from build123d import *

# Parameters (mm, degrees)
SKETCH_1_R          = 1.25
SKETCH_1_R_2        = 4.8
EXTRUDE_1_DEPTH     = 2
SKETCH_3_R          = 6.5
SKETCH_3_R_2        = 4.8
EXTRUDE_2_DEPTH     = 2
SKETCH_5_R          = 1.25
CUT_EXTRUDE_1_DEPTH = 10


with BuildPart() as part:
    # 草图1 → 凸台-拉伸1 (new body)
    with BuildSketch(Plane(origin=(0, 0, 0), x_dir=(1, 0, 0), z_dir=(0, 1, 0))):
        with BuildLine():
            Line((10.5, -13.247031622), (-10.5, -13.247031622))
            ThreePointArc((-10.5, -13.247031622), (-14.742640687, -11.489672309), (-16.5, -7.247031622))
            Line((-16.5, -7.247031622), (-16.5, 7.247031622))
            ThreePointArc((-16.5, 7.247031622), (-14.742640687, 11.489672309), (-10.5, 13.247031622))
            Line((-10.5, 13.247031622), (10.5, 13.247031622))
            ThreePointArc((10.5, 13.247031622), (14.742640687, 11.489672309), (16.5, 7.247031622))
            Line((16.5, 7.247031622), (16.5, -7.247031622))
            ThreePointArc((16.5, -7.247031622), (14.742640687, -11.489672309), (10.5, -13.247031622))
        make_face()
        with Locations(Location((0, 8, 0), (0, 0, 270))):
            Circle(SKETCH_1_R, mode=Mode.SUBTRACT)
        with Locations(Location((0, -8, 0), (0, 0, 270))):
            Circle(SKETCH_1_R, mode=Mode.SUBTRACT)
        with Locations(Location((-9.5, 0, 0), (0, 0, 270))):
            Circle(SKETCH_1_R, mode=Mode.SUBTRACT)
        with Locations(Location((9.5, 0, 0), (0, 0, 270))):
            Circle(SKETCH_1_R, mode=Mode.SUBTRACT)
        with Locations(Location((0, 0, 0), (0, 0, 270))):
            Circle(SKETCH_1_R_2, mode=Mode.SUBTRACT)
    extrude(amount=EXTRUDE_1_DEPTH)

    # 草图3 → 凸台-拉伸2 (add)
    with BuildSketch(Plane(origin=(0, 2, 0), x_dir=(1, 0, 0), z_dir=(0, 1, 0))):
        with Locations(Location((0, 0, 0), (0, 0, 90))):
            Circle(SKETCH_3_R)
        with Locations(Location((0, 0, 0), (0, 0, 270))):
            Circle(SKETCH_3_R_2, mode=Mode.SUBTRACT)
    extrude(amount=EXTRUDE_2_DEPTH)

    # 草图5 → 切除-拉伸1 (cut)
    with BuildSketch(Plane(origin=(0, 2, 0), x_dir=(1, 0, 0), z_dir=(0, 1, 0))):
        with Locations(Location((-12.23, 2.77, 0), (0, 0, 270))):
            Circle(SKETCH_5_R)
        with Locations(Location((-12.23, -2.77, 0), (0, 0, 270))):
            Circle(SKETCH_5_R)
        with Locations(Location((12.23, -2.77, 0), (0, 0, 270))):
            Circle(SKETCH_5_R)
        with Locations(Location((12.23, 2.77, 0), (0, 0, 270))):
            Circle(SKETCH_5_R)
    extrude(amount=-CUT_EXTRUDE_1_DEPTH, mode=Mode.SUBTRACT)


solid = part.part
Source: CAD feature listing. Evaluate the final solid. Frame: model axes, mm. Coordinates: 2 decimals unless noted, no trailing zeros. Order: outer loops, then holes, each group sorted by start corner. A loop starts at its lowest first (then second) coordinate and runs counter-clockwise, first axis right, second up.
Item 1: Material intervals for line 1 (X direction, y = 1.2, z = 0); line 2 (X direction, y = 0.9, z = 2.77); line 3 (Y direction, x = 13, z = -7.25), sorted ascending.
Output values:
line 1: x = -16.5 to -10.75, -8.25 to -4.8, 4.8 to 8.25, 10.75 to 16.5
line 2: x = -16.5 to -13.48, -10.98 to -3.92, 3.92 to 10.98, 13.48 to 16.5
line 3: y = 0 to 2
Item 2: Cut plane B-B (z = 0). Return loops of the section in (x, y), plus the area to 3 significant figures.
Output values:
outline: (-16.5, 0) - (-10.75, 0) - (-10.75, 2) - (-16.5, 2) - close; (-8.25, 0) - (-4.8, 0) - (-4.8, 4) - (-6.5, 4) - (-6.5, 2) - (-8.25, 2) - close; (4.8, 0) - (8.25, 0) - (8.25, 2) - (6.5, 2) - (6.5, 4) - (4.8, 4) - close; (10.75, 0) - (16.5, 0) - (16.5, 2) - (10.75, 2) - close
area: 43.6 mm2
Item 3: Pull-direction query (X, two-part tool) for faces 1 (the face through (-3, 2, 6)), 2 (the face through (14.79, 0.99, 11.44)), 3 (the face through (-8.26, 0.99, -0.16)); classes: pulls with the +X half, pulls with the -X half, needs draft (parallel to the pull), parting line crosses it, or undercut.
Output values:
face 1: needs draft
face 2: pulls with the +X half
face 3: undercut
Item 4: First-contact query: P1, Ø2, axis at x = 0, z = 8, coming from the +Y side; P2, Ø2, axis at y = 1.5, z = -10, coming from the +X side; P3, Ø1, axis at y = 1, z = 8, coming from the +X side; P4, Ø1.5, axis at x = -12, z = 8, coming from the +Y side. Flat tips, straight axial feed; report the tip coordinate or a pass-through.
Output values:
P1: passes through
P2: stops at x = 16.24
P3: stops at x = 16.49
P4: stops at y = 2
Item 5: Cut plane C-C (x = -6). Return loops of the section in (y, z).
Output values:
outline: (0, -13.25) - (2, -13.25) - (2, -2.5) - (4, -2.5) - (4, 2.5) - (2, 2.5) - (2, 13.25) - (0, 13.25) - close
Item 6: Cut plane D-D (z = -8). Return loops of the section in (x, y), plus the area to 3 significant figures.
Output values:
outline: (-16.45, 0) - (-1.25, 0) - (-1.25, 2) - (-16.45, 2) - close; (1.25, 0) - (16.45, 0) - (16.45, 2) - (1.25, 2) - close
area: 60.8 mm2
Item 7: Cut plane A-A (x = 9.5). Return loops of the section in (y, z), plus the area to 3 significant figures.
Output values:
outline: (0, -13.25) - (2, -13.25) - (2, -1.25) - (0, -1.25) - close; (0, 1.25) - (2, 1.25) - (2, 13.25) - (0, 13.25) - close
area: 48.0 mm2
